Could you check a few things on this model? Use its own coordinates, in mm. A direction names the side the tool comes from. Round coordinates to 2 decimals unless told otherwise and drop trailing zeros. Loops run counter-clockwise (first coordinate to the right, second up) from the corner with the lowest first, then second, coordinate; pieces in that order, holes last. Notation, with made-up numbers: (59.5, -36.5) -> (83.5, -36.5) arc R16 ccw to (83.5, -26.5) -> close; hole circle Ø1 at (54, 60.5). An arc over 180 degrees is marked (long way). One line per item, written item: value.
```python
from build123d import *

# Parameters (mm, degrees)
SKETCH_1_R          = 100
EXTRUDE_1_DEPTH     = 19
M6X1_0_1_D          = 5
M6X1_0_1_DEPTH      = 17
M6X1_0_1_TIP        = 1.502151548
SKETCH_2_R          = 8
CUT_EXTRUDE_1_DEPTH = 143.691975948
CHAMFER_1_SIZE      = 1
CHAMFER_2_SIZE      = 1


with BuildPart() as part:
    # ｽｹｯﾁ1 → ﾎﾞｽ - 押し出し1 (new body)
    with BuildSketch(Plane.XY):
        Circle(SKETCH_1_R)
    extrude(amount=EXTRUDE_1_DEPTH)

    # M6x1.0 ねじ穴1
    with Locations(Plane(origin=(0, 90, 19), x_dir=(1, 0, 0), z_dir=(0, 0, 1))):
        with Locations((0, 0), (-90, -90), (0, -180), (90, -90)):
            Hole(M6X1_0_1_D / 2, depth=M6X1_0_1_DEPTH)
            with Locations((0, 0, -(M6X1_0_1_DEPTH + M6X1_0_1_TIP / 2))):  # 118° drill point
                Cone(0, M6X1_0_1_D / 2, M6X1_0_1_TIP, mode=Mode.SUBTRACT)

    # ｽｹｯﾁ2 → ｶｯﾄ - 押し出し1 (cut, through all)
    with BuildSketch(Plane.XY.offset(19)):
        Circle(SKETCH_2_R)
    extrude(amount=-CUT_EXTRUDE_1_DEPTH, mode=Mode.SUBTRACT)

    # 面取り1
    chamfer_1_edges = [part.edges().sort_by_distance(p)[0] for p in [
        (-8, 0, 19),
    ]]
    chamfer(chamfer_1_edges, length=CHAMFER_1_SIZE)

    # 面取り2
    chamfer_2_edges = [part.edges().sort_by_distance(p)[0] for p in [
        (-8, 0, 0),
    ]]
    chamfer(chamfer_2_edges, length=CHAMFER_2_SIZE)


solid = part.part
```
(1) Imagine slicing it at C-C on y = 32. Write out the boundary of the cut face in (x, z).
Results below:
outline: (-94.74, 0) -> (94.74, 0) -> (94.74, 19) -> (-94.74, 19) -> close
(2) Please list where these lines run through material, in increasing order: L1, parallel to Y at x = 0, z = 13.75; L2, parallel to Y at x = 90, z = 12.5.
Results below:
L1: y = -100 to -92.5, -87.5 to -8, 8 to 87.5, 92.5 to 100
L2: y = -43.59 to -2.5, 2.5 to 43.59
(3) On a 3-axis mill with a long thin cutter (end or side, diameter ignored), from which of +Z, -Z, +X, -X, +Y, -Y can I reach the whole of each face in a straight line? I mean faces 4 (the face through (92.5, 0.1, 10.4)), 5 (the face through (-1, -21, 0)). Say none if no direction works.
Results below:
face 4: +Z
face 5: -Z, +X, -X, +Y, -Y
(4) Imagine slicing it at A-A on z = 15. Write out the boundary of the cut face in (x, y), then the cut area to 3 significant figures.
Results below:
outline: circle Ø200 at (0, 0); hole circle Ø5 at (-90, 0); hole circle Ø16 at (0, 0); hole circle Ø5 at (0, -90); hole circle Ø5 at (0, 90); hole circle Ø5 at (90, 0)
area: 31,100 mm²
(5) Imagine slicing it at B-B on x = 60. Write out the boundary of the cut face in (y, z), then the cut area to 3 significant figures.
Results below:
outline: (-80, 0) -> (80, 0) -> (80, 19) -> (-80, 19) -> close
area: 3,040 mm²
(6) We'd pull the mould along Y, two halves only. Please class faces 1 (the face through (-0.06, -89.57, 0.76)), 2 (the face through (95.38, 30.04, 9.37)), 3 (the face through (-1, -21, 19)): +Y half, -Y half, draft (parallel to the pull), parting line (faces both ways), or undercut.
Results below:
face 1: undercut
face 2: parting line
face 3: draft
(7) For pin 1 Ø8 at (y, z) = (46.5, 3.5) entering from +X; pin 2 Ø4 at (y, z) = (-10, 5.5) entering from +X; pin 3 Ø1 at (y, z) = (56, 15.5) entering from -X; pin 4 Ø13 at (x, y) = (0, 0) entering from +Z, each with a flat end and sliding along its axis, tell me the tip position at first contact or that it passes through.
Results below:
pin 1: stops at x = 90.52
pin 2: stops at x = 99.68
pin 3: stops at x = -83.19
pin 4: passes through
